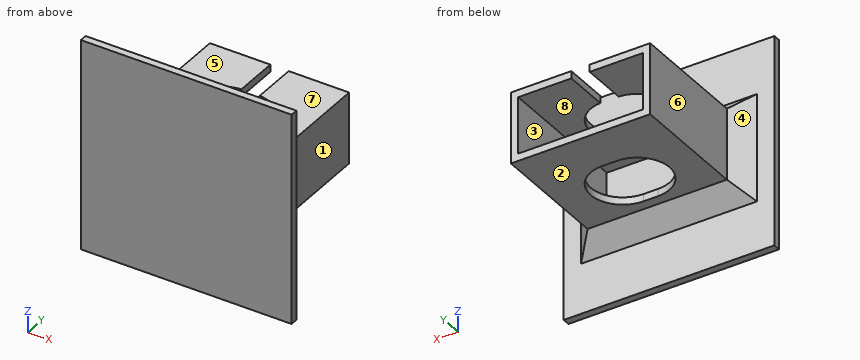
```python
from build123d import *

# Parameters (mm, degrees)
SKETCH1_W           = 76
SKETCH1_H           = 39
SKETCH1_W_2         = 68
SKETCH1_H_2         = 31
BOSS_EXTRUDE2_DEPTH = 75
SKETCH1_9_W         = 115
SKETCH1_9_H         = 115
SKETCH1_9_W_2       = 76
SKETCH1_9_H_2       = 39
SKETCH1_9_W_3       = 68
SKETCH1_9_H_3       = 31
BOSS_EXTRUDE6_DEPTH = 4
SKETCH9_W           = 10
SKETCH9_H           = 75
CUT_EXTRUDE2_DEPTH  = 6
CUT_EXTRUDE3_DEPTH  = 52
CHAMFER1_SIZE       = 10


with BuildPart() as part:
    # Sketch1 → Boss-Extrude2 (new body)
    with BuildSketch(Plane(origin=(0, 0, 0), x_dir=(1, 0, 0), z_dir=(0, 1, 0))):
        with Locations((34, 15.5)):
            Rectangle(SKETCH1_W, SKETCH1_H)
        with Locations((34, 15.5)):
            Rectangle(SKETCH1_W_2, SKETCH1_H_2, mode=Mode.SUBTRACT)
    extrude(amount=BOSS_EXTRUDE2_DEPTH)

    # Sketch1_9 → Boss-Extrude6 (add)
    # profile 1 of 3: a face of its own
    with BuildSketch(Plane(origin=(0, 0, 0), x_dir=(1, 0, 0), z_dir=(0, 1, 0))):
        with Locations((34, 15)):
            Rectangle(SKETCH1_9_W, SKETCH1_9_H)
        with Locations((34, 15.5)):
            Rectangle(SKETCH1_9_W_2, SKETCH1_9_H_2, mode=Mode.SUBTRACT)
    # profile 2 of 3: a face of its own
    with BuildSketch(Plane(origin=(0, 0, 0), x_dir=(1, 0, 0), z_dir=(0, 1, 0))):
        with Locations((34, 15.5)):
            Rectangle(SKETCH1_9_W_2, SKETCH1_9_H_2)
        with Locations((34, 15.5)):
            Rectangle(SKETCH1_9_W_3, SKETCH1_9_H_3, mode=Mode.SUBTRACT)
    # profile 3 of 3: a face of its own
    with BuildSketch(Plane(origin=(0, 0, 0), x_dir=(1, 0, 0), z_dir=(0, 1, 0))):
        with Locations((34, 15.5)):
            Rectangle(SKETCH1_9_W_3, SKETCH1_9_H_3)
    extrude(amount=-BOSS_EXTRUDE6_DEPTH)

    # Sketch9 → Cut-Extrude2 (cut)
    with BuildSketch(Plane.XY.offset(4)):
        with Locations((34, 37.5)):
            Rectangle(SKETCH9_W, SKETCH9_H)
    extrude(amount=-CUT_EXTRUDE2_DEPTH, mode=Mode.SUBTRACT)

    # Sketch7 → Cut-Extrude3 (cut)
    with BuildSketch(Plane.XY.offset(4)):
        with BuildLine():
            Line((30, 50.5), (38, 50.5))
            ThreePointArc((38, 50.5), (55.5, 33), (38, 15.5))
            Line((38, 15.5), (30, 15.5))
            ThreePointArc((30, 15.5), (12.5, 33), (30, 50.5))
        make_face()
    extrude(amount=-CUT_EXTRUDE3_DEPTH, mode=Mode.SUBTRACT)

    # Chamfer1
    chamfer1_edges = [part.edges().sort_by_distance(p)[0] for p in [
        (55.5, 0, 4),
        (12.5, 0, 4),
        (72, 0, -15.5),
        (34, 0, -35),
        (-4, 0, -15.5),
    ]]
    chamfer(chamfer1_edges, length=CHAMFER1_SIZE)


solid = part.part
```
Part model, mm, in its own coordinate system. Face numbers are marked on the shaded views. A direction names the side the tool comes from. Round coordinates to 2 decimals unless told otherwise and drop trailing zeros. Loops run counter-clockwise (first coordinate to the right, second up) from the corner with the lowest first, then second, coordinate; pieces in that order, holes last. Notation, with made-up numbers: (50.5, 9.5) -> (59.5, 9.5) arc R19 ccw to (59.5, 26.5) -> close; hole circle Ø5 at (46, -21). An arc over 180 degrees is marked (long way). Use one line per item in the form item = value. Start each with the question number.
Item 1: Drop flat-ended pins along their axis: pin 1 Ø3 at (x, z) = (20.5, -47.5) entering from +Y; pin 2 Ø14.5 at (x, y) = (50.5, 29.5) entering from -Z; pin 3 Ø6 at (y, z) = (6, -10.5) entering from +X. Give the stop position or say it passes through.
Item 2: Band-saw the part on C-C (z = -33). List the corners of the cut face in (x, y).
Item 3: Band-saw the part on A-A (y = 33). List the corners of the cut face in (x, z), plus the area to 3 significant figures.
Item 4: Two-plate mould, pull along X, no slides. Class the marked faces 6, 7 and 8: released by +X, released by -X, zero draft, split by the parting line, or undercut.
Item 5: Tool access for the marked faces 1, 2, 3, 4 and 5: list every direction of +Z, -Z, +X, -X, +Y, -Y with a clear straight run to the whole face (end or side of a thin tool).
Item 6: Band-saw the part on D-D (x = -7). List the corners of the cut face in (y, z).
Item 7: Drill centre lines: line 1 along Z through (x, y) = (8.5, 59); line 2 along Y through (x, z) = (-17.5, -12); line 3 along Z through (x, y) = (59, 4.5). Where is each one in solid material? Low to high.
Item 8: Band-saw the part on B-B (x = 51). List the corners of the cut face in (y, z), plus the area to 3 significant figures.
Data:
q1.pin_1 = 0
q1.pin_2 = -35
q1.pin_3 = 79
q2.outline = (-23.5, -4) -> (91.5, -4) -> (91.5, 0) -> (82, 0) -> (72, 10) -> (72, 75) -> (-4, 75) -> (-4, 10) -> (-14, 0) -> (-23.5, 0) -> close; hole (30, 15.5) -> (38, 15.5) arc R17.5 ccw to (38, 50.5) -> (30, 50.5) arc R17.5 ccw to start
q3.outline = (-4, -35) -> (12.5, -35) -> (12.5, -31) -> (0, -31) -> (0, 0) -> (12.5, 0) -> (12.5, 4) -> (-4, 4) -> close; (55.5, -35) -> (72, -35) -> (72, 4) -> (55.5, 4) -> (55.5, 0) -> (68, 0) -> (68, -31) -> (55.5, -31) -> close
q3.area = 512 mm^2
q4.face_6 = released by -X
q4.face_7 = zero draft
q4.face_8 = undercut
q5.face_1 = +Z, -Z, +X, +Y
q5.face_2 = -Z, +X, -X, +Y
q5.face_3 = +Y
q5.face_4 = +Z, -Z, -X, +Y
q5.face_5 = +Z, +X, -X, +Y
q6.outline = (-4, -72.5) -> (0, -72.5) -> (0, -45) -> (7, -38) -> (7, 7) -> (0, 14) -> (0, 42.5) -> (-4, 42.5) -> close
q7.line_1 = -35 to -31, 0 to 4
q7.line_2 = -4 to 0
q7.line_3 = -40.5 to -31, 0 to 9.5
q8.outline = (-4, -72.5) -> (0, -72.5) -> (0, -45) -> (10, -35) -> (21.28, -35) -> (21.28, -31) -> (0, -31) -> (0, 0) -> (21.28, 0) -> (21.28, 4) -> (10, 4) -> (0, 14) -> (0, 42.5) -> (-4, 42.5) -> close; (44.72, -35) -> (75, -35) -> (75, -31) -> (44.72, -31) -> close; (44.72, 0) -> (75, 0) -> (75, 4) -> (44.72, 4) -> close
q8.area = 973 mm^2
